from build123d import *

# Parameters (mm, degrees)
BASE_FLANGE1_DEPTH                 = 35
SKETCH10_W                         = 28
SKETCH10_H                         = 14
CUT_EXTRUDE1_DEPTH                 = 4
F_4_0_4_DIAMETER_HOLE1_D           = 4
F_4_0_4_DIAMETER_HOLE1_CSINK_D     = 4.05
F_4_0_4_DIAMETER_HOLE1_CSINK_ANGLE = 90
SCALE1_SCALE                       = 1.5
CUT_EXTRUDE2_DEPTH                 = 10
CUT_EXTRUDE3_DEPTH                 = 10
FILLET1_R                          = 1.5


# Sheet-metal steps are written as plain solids
with BuildPart() as part:
    # Sketch1 → Base-Flange1 (new body)
    with BuildSketch(Plane.XY):
        with BuildLine():
            Line((0, 0), (-9, 0))
            ThreePointArc((-9, 0), (-11.121320344, 0.878679656), (-12, 3))
            Line((-12, 3), (-12, 15))
            ThreePointArc((-12, 15), (-12.292893219, 15.707106781), (-13, 16))
            Line((-13, 16), (-35, 16))
            ThreePointArc((-35, 16), (-35.707106781, 15.707106781), (-36, 15))
            Line((-36, 15), (-36, 3))
            ThreePointArc((-36, 3), (-36.878679656, 0.878679656), (-39, 0))
            Line((-39, 0), (-48, 0))
            Line((-48, 0), (-48, 2))
            Line((-48, 2), (-39, 2))
            ThreePointArc((-39, 2), (-38.292893219, 2.292893219), (-38, 3))
            Line((-38, 3), (-38, 15))
            ThreePointArc((-38, 15), (-37.121320344, 17.121320344), (-35, 18))
            Line((-35, 18), (-13, 18))
            ThreePointArc((-13, 18), (-10.878679656, 17.121320344), (-10, 15))
            Line((-10, 15), (-10, 3))
            ThreePointArc((-10, 3), (-9.707106781, 2.292893219), (-9, 2))
            Line((-9, 2), (0, 2))
            Line((0, 2), (0, 0))
        make_face()
    extrude(amount=-BASE_FLANGE1_DEPTH)

    # Sketch10 → Cut-Extrude1 (cut)
    with BuildSketch(Plane(origin=(0, 18, 0), x_dir=(1, 0, 0), z_dir=(0, 1, 0))):
        with Locations((-24, 7)):
            Rectangle(SKETCH10_W, SKETCH10_H)
    extrude(amount=-CUT_EXTRUDE1_DEPTH, mode=Mode.SUBTRACT)

    # Ø4.0 (4) Diameter Hole1 (through all)
    with Locations(Plane(origin=(0, 18, 0), x_dir=(1, 0, 0), z_dir=(0, 1, 0))):
        with Locations((-24, 27), (-24, 19), (-43, 30), (-43, 5), (-5, 30), (-5, 5)):
            CounterSinkHole(F_4_0_4_DIAMETER_HOLE1_D / 2, F_4_0_4_DIAMETER_HOLE1_CSINK_D / 2, counter_sink_angle=F_4_0_4_DIAMETER_HOLE1_CSINK_ANGLE)


with BuildPart() as part_1:
    # Scale1: scaled about (-24, 8.107482912, -19.478199083)
    add(part.part.scale(SCALE1_SCALE).moved(Location((12, -4.053741456, 9.739099541))))

    # Sketch15 → Cut-Extrude2 (cut)
    with BuildSketch(Plane(origin=(0, -1.053741456, 0), x_dir=(1, 0, 0), z_dir=(0, 1, 0))):
        with BuildLine():
            Line((-60, 38.767251784), (-60, 42.760900459))
            Line((-60, 42.760900459), (-56.006351326, 42.760900459))
            ThreePointArc((-56.006351326, 42.760900459), (-58.830287385, 41.591187844), (-60, 38.767251784))
        make_face()
        with BuildLine():
            Line((-60, -9.739099541), (-56.006351326, -9.739099541))
            ThreePointArc((-56.006351326, -9.739099541), (-58.830287385, -8.569386926), (-60, -5.745450867))
            Line((-60, -5.745450867), (-60, -9.739099541))
        make_face()
        with BuildLine():
            Line((12, -5.745450867), (12, -9.739099541))
            Line((12, -9.739099541), (8.006351326, -9.739099541))
            ThreePointArc((8.006351326, -9.739099541), (10.830287385, -8.569386926), (12, -5.745450867))
        make_face()
        with BuildLine():
            Line((12, 42.760900459), (8.006351326, 42.760900459))
            ThreePointArc((8.006351326, 42.760900459), (10.830287385, 41.591187844), (12, 38.767251784))
            Line((12, 38.767251784), (12, 42.760900459))
        make_face()
    extrude(amount=-CUT_EXTRUDE2_DEPTH, mode=Mode.SUBTRACT)

    # Sketch16 → Cut-Extrude3 (cut)
    with BuildSketch(Plane(origin=(0, -1.053741456, 0), x_dir=(1, 0, 0), z_dir=(0, 1, 0))):
        with BuildLine():
            Line((-54.703281617, 24.816516721), (-59.364976604, 30.038451214))
            ThreePointArc((-59.364976604, 30.038451214), (-59.835855465, 30.812399385), (-60, 31.703342281))
            Line((-60, 31.703342281), (-60, 1.311607043))
            ThreePointArc((-60, 1.311607043), (-59.839618442, 2.192620974), (-59.379051563, 2.960596195))
            Line((-59.379051563, 2.960596195), (-54.698537483, 8.165669485))
            ThreePointArc((-54.698537483, 8.165669485), (-54.186063754, 9.006077869), (-54, 9.972667676))
            Line((-54, 9.972667676), (-54, 22.972667676))
            ThreePointArc((-54, 22.972667676), (-54.181788316, 23.959377402), (-54.703281617, 24.816516721))
        make_face()
        with BuildLine():
            Line((11.364976604, 30.038451214), (6.703281617, 24.816516721))
            ThreePointArc((6.703281617, 24.816516721), (6.181788316, 23.959377402), (6, 22.972667676))
            Line((6, 22.972667676), (6, 9.972667676))
            ThreePointArc((6, 9.972667676), (6.186063754, 9.006077869), (6.698537483, 8.165669485))
            Line((6.698537483, 8.165669485), (11.379051563, 2.960596195))
            ThreePointArc((11.379051563, 2.960596195), (11.839618442, 2.192620974), (12, 1.311607043))
            Line((12, 1.311607043), (12, 31.703342281))
            ThreePointArc((12, 31.703342281), (11.835855465, 30.812399385), (11.364976604, 30.038451214))
        make_face()
    extrude(amount=-CUT_EXTRUDE3_DEPTH, mode=Mode.SUBTRACT)

    # Fillet1
    fillet1_edges = [part_1.edges().sort_by_distance(p)[0] for p in [
        (-3, 16.946258544, -0.760900459),
        (-45, 16.946258544, -0.760900458),
        (-6, 16.946258544, -0.760900459),
        (-42, 16.946258544, -0.760900459),
    ]]
    fillet(fillet1_edges, radius=FILLET1_R - 0.0001)  # a hair under: the kernel refuses the full size

    # Sketch18 → Revolve1 (revolve)
    with BuildSketch(Plane(origin=(0, 0, -30.760900459), x_dir=(-1, 0, 0), z_dir=(0, 0, -1)), mode=Mode.PRIVATE) as revolve1_sk:
        with BuildLine():
            Line((27, 19.946258544), (27, 17.298747157))
            ThreePointArc((27, 17.298747157), (27.231953871, 17.32602037), (27.451255487, 17.406352354))
            Line((27.451255487, 17.406352354), (29.130617451, 19.638600901))
            ThreePointArc((29.130617451, 19.638600901), (29.402592072, 19.865072033), (29.747074465, 19.946258544))
            Line((29.747074465, 19.946258544), (27, 19.946258544))
        make_face()
    revolve(revolve1_sk.sketch.rotate(Axis((-24, 22.908758544, -30.760900459), (0, -1, 0)), 270), axis=Axis((-24, 22.908758544, -30.760900459), (0, -1, 0)))

    # Sketch20 → Revolve2 (revolve)
    with BuildSketch(Plane(origin=(0, 0, -18.760900459), x_dir=(-1, 0, 0), z_dir=(0, 0, -1)), mode=Mode.PRIVATE) as revolve2_sk:
        with BuildLine():
            Line((29.747074465, 19.946258544), (27, 19.946258544))
            Line((27, 19.946258544), (27, 17.298747157))
            ThreePointArc((27, 17.298747157), (27.231953871, 17.32602037), (27.451255487, 17.406352354))
            Line((27.451255487, 17.406352354), (29.130617451, 19.638600901))
            ThreePointArc((29.130617451, 19.638600901), (29.402592072, 19.865072033), (29.747074465, 19.946258544))
        make_face()
    revolve(revolve2_sk.sketch.rotate(Axis((-24, 19.946258544, -18.760900459), (0, 1, 0)), 270), axis=Axis((-24, 19.946258544, -18.760900459), (0, 1, 0)))


solid = part_1.part
Work out the finished part from the listing and answer in its coordinate system (mm). A direction names the side the tool comes from. Give positions to 0.01 mm unless a question says otherwise; leave off trailing zeros. Loops run counter-clockwise (first coordinate to the right, second up) from the corner with the lowest first, then second, coordinate; pieces in that order, holes last. Notation, with made-up numbers: (64, -26) - (80, -26) arc R17 ccw to (80, -11) - close; hole circle Ø11 at (4, -10.5). An arc over 180 degrees is marked (long way). Answer in a Markdown table with one row per item. Add a question column.
Q1. A tool of negligible diameter and unlimited length cuts with its end or side. For faces 1 (the flat face through (6, -3, -17)), 2 (the flat face through (-57.07, -2.53, -5.53)), 3 (the flat face through (-45, 9, -16)), 4 (the cylindrical face through (-26.645, 19.441, -29.346)), 5 (the cylindrical face through (-44.57, 16.5, -0.91)), from which of +Z, -Z, +X, -X, +Y, -Y can it reach the whole face along a straight path? Write none if from no direction.
Q2. The part is cut by section A-A (x = 4.5). Determine the outline of the cut face in (y, z).
Q3. The part is cut by section C-C (x = -24). Determine the outline of the cut face in (y, z), and give its area (3 significant figures).
Q4. The part is cut by section D-D (x = -11). Determine the outline of the cut face in (y, z).
Q5. Consider line 1 along Z through (x, y) = (-52.5, -2.5); line 2 along Z through (x, y) = (-24, 21.7); line 3 along X through (y, z) = (0.5, -25.5). Determine where each line is inside the solid, lowest interval first.
Q6. Determine the mould class of faces 6 (the cylindrical face through (-4.35, 21.66, -26.79)), 7 (the flat face through (-60, -3, -35)), 8 (the cylindrical face through (-26.645, 19.441, -20.176)) for opening direction X: released by +X, released by -X, zero draft, split by the parting line, or undercut.
Q7. Each of these flat-tipped pins is pushed along its axis until it touches: P1, Ø6, axis at x = -3.5, z = -13.5, coming from the -Y side; P2, Ø7, axis at x = -24, z = -30.76, coming from the -Y side; P3, Ø3, axis at x = 2, z = -36, coming from the +Y side; P4, Ø10, axis at x = -11.5, z = -30, coming from the -Y side. Where does it stop, or does it pass through?
Solution:
| question | item | result |
|---|---|---|
| 1 | face 1 | +X, +Y, -Y |
| 1 | face 2 | -X, +Y, -Y |
| 1 | face 3 | +Z, -Z, -X, +Y |
| 1 | face 4 | +Y, -Y |
| 1 | face 5 | +Z, -X, +Y |
| 2 | outline | (-4.05, -42.76) - (-1.05, -42.76) - (-1.05, -38.26) - (-4.05, -38.26) - close; (-4.05, -32.26) - (-1.05, -32.26) - (-1.05, -0.76) - (-4.05, -0.76) - close; (-4.05, 5.24) - (-1.05, 5.24) - (-1.05, 9.74) - (-4.05, 9.74) - close |
| 3 | outline | (17.3, -33.76) arc R1 ccw to (17.41, -34.21) - (19.64, -35.89) arc R0.77 cw to (19.95, -36.51) - (19.95, -42.76) - (22.95, -42.76) - (22.95, -33.8) - (22.91, -33.76) - close; (17.3, -27.76) - (22.91, -27.76) - (22.95, -27.72) - (22.95, -21.8) - (22.91, -21.76) - (17.3, -21.76) arc R1 ccw to (17.41, -22.21) - (19.64, -23.89) arc R0.77 cw to (19.95, -24.51) - (19.95, -25.01) arc R0.77 cw to (19.64, -25.63) - (17.41, -27.31) arc R1 ccw to start; (17.3, -15.76) - (22.91, -15.76) - (22.95, -15.72) - (22.95, -11.26) - (19.95, -11.26) - (19.95, -13.01) arc R0.77 cw to (19.64, -13.63) - (17.41, -15.31) arc R1 ccw to start |
| 3 | area | 73.0 mm² |
| 4 | outline | (19.95, -42.76) - (22.95, -42.76) - (22.95, -11.26) - (19.95, -11.26) - close |
| 5 | line 1 | z = -42.76 to -38.26, -32.26 to -0.76, 5.24 to 9.74 |
| 5 | line 2 | z = -42.76 to -33.76, -27.76 to -21.76, -15.76 to -11.26 |
| 5 | line 3 | x = -45 to -42, -6 to -3 |
| 6 | face 6 | released by +X |
| 6 | face 7 | released by -X |
| 6 | face 8 | undercut |
| 7 | P1 | stops at y = -4.05 |
| 7 | P2 | stops at y = 17.3 |
| 7 | P3 | stops at y = -1.05 |
| 7 | P4 | stops at y = 19.56 |
